Drawing for the job (mm, zero at the part's lowest x, y, z). Coordinates: 2 decimals unless noted, no trailing zeros. Write each loop counter-clockwise with the first axis right and the second up, starting at its lowest first coordinate (ties: lowest second). Pieces come first, ordered by that corner, then holes. Notation, with made-up numbers: M 43,63.5 L 59,63.5 A22 ccw 59,71.5 Z; hole C 77.25,52 d1. An arc over 180 degrees is marked long. Put each result on its own line as item: value. Start each with the question number.
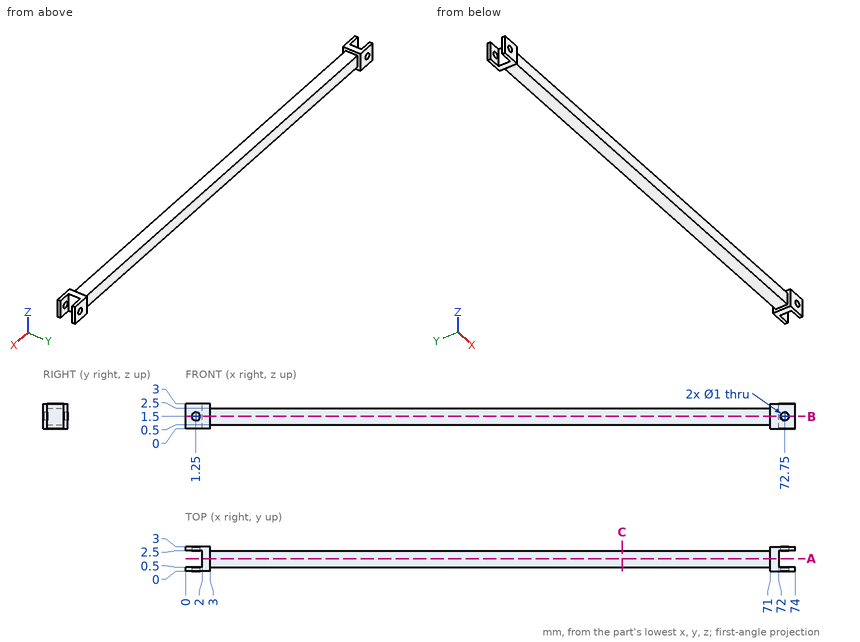
(1) Slice it at A-A, the plane y = 1.55. Write the cut outline in (x, z).
(2) Drill centre lines: line 1 (Z direction, x = 1.25, y = 2.7); line 2 (X direction, y = 1.8, z = 2.85); line 3 (X direction, y = 0.3, z = 2.7). Where is each one in solid material? Low to high. Write a range as [from, to].
(3) Drop flat-ended pins along their axis: pin 1 (0.6 mm diameter, centred on y = 1.5, z = 1.5, fed in from +X); pin 2 (1 mm diameter, centred on x = 28.5, y = 1, fed in from +Z); pin 3 (1 mm diameter, centred on x = 42.5, y = 1.5, fed in from -Z). Give the stop position or say it passes through.
(4) Slice it at B-B, the plane z = 1.5. State how many separate pieces and enclosed holes the cut face has, then the cut area to 3 significant figures.
(5) Slice it at C-C, the plane x = 53. Write the cut outline in (y, z).
Result set:
1. outline: M 2,0 L 3,0 L 3,0.5 L 71,0.5 L 71,0 L 72,0 L 72,3 L 71,3 L 71,2.5 L 3,2.5 L 3,3 L 2,3 Z
2. line 1: z = [0, 1], [2, 3]
2. line 2: x = [2, 3], [71, 72]
2. line 3: x = [0, 3], [71, 74]
3. pin 1: stops at x = 72
3. pin 2: stops at z = 2.5
3. pin 3: stops at z = 0.5
4. separate pieces: 5
4. enclosed holes: 0
4. area: 144 mm^2
5. outline: M 0.5,0.5 L 2.5,0.5 L 2.5,2.5 L 0.5,2.5 Z
